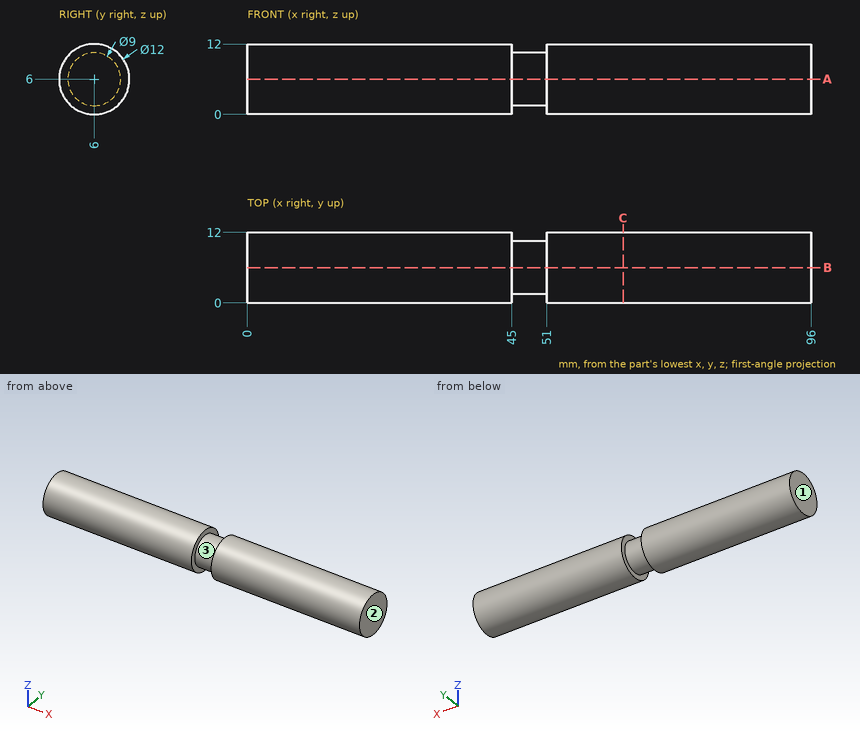
Could you check a few things on this drawing? It's one solid part, dimensions in mm from its lowest x, y, z. Round coordinates to 2 decimals unless told otherwise and drop trailing zeros. Loops run counter-clockwise (first coordinate to the right, second up) from the corner with the lowest first, then second, coordinate; pieces in that order, holes last. Notation, with made-up numbers: M -28,14 L 0,14 A20 ccw 0,39 Z; hole C 81,-19.75 d7. An arc over 180 degrees is marked long. Write item = value, one per line. Start each with the question number.
(1) If we mould it in two halves opening along X, with no side actions, what happens to the marked faces 1, 2 and 3? For each: released by +X, released by -X, zero draft, split by the parting line, or undercut.
(2) I'm going to push flat-ended pins straight in: P1, Ø2, axis at x = 52.5, y = 9, coming from the +Z side; P2, Ø2, axis at x = 33.5, y = 10.5, coming from the -Z side; P3, Ø1, axis at x = 22, z = 8, coming from the -Y side. Where does each tip first touch, or does it pass through?
(3) Suppose I cut it at A-A on z = 6. Write out the boundary of the cut face in (x, y).
(4) I need wall thicknesses on line 1 along X through (y, z) = (0.75, 3.25); line 2 along Y through (x, z) = (82.5, 6.25); line 3 along Z through (x, y) = (30, 9). Which ranges of each line are inside material? Lowest first, please.
(5) Suppose I cut it at C-C on x = 64. Write out the boundary of the cut face in (y, z), plus the area to 3 significant figures.
Answer block:
q1.face_1 = released by -X
q1.face_2 = released by +X
q1.face_3 = undercut
q2.P1 = 11.66
q2.P2 = 1.13
q2.P3 = 0.19
q3.outline = M 0,0 L 45,0 L 45,1.5 L 51,1.5 L 51,0 L 96,0 L 96,12 L 51,12 L 51,10.5 L 45,10.5 L 45,12 L 0,12 Z
q4.line_1 = 0 to 45, 51 to 96
q4.line_2 = 0.01 to 11.99
q4.line_3 = 0.8 to 11.2
q5.outline = C 6,6 d12
q5.area = 113 mm²
